Verification items for the finished model (mm, model axes). Face numbers are marked on the shaded views. Round coordinates to 2 decimals unless told otherwise and drop trailing zeros. Write each loop counter-clockwise with the first axis right and the second up, starting at its lowest first coordinate (ties: lowest second). Pieces come first, ordered by that corner, then holes. Notation, with made-up numbers: (0, 29.25) -> (19, 29.25) arc R27 cw to (19, 68.25) -> close; hole circle Ø8 at (89, 8.25). An arc over 180 degrees is marked (long way). Answer as a JSON object with one key per item and string values. Group by question number.
(1) Sectioned sample at A-A on z = 5.5. Record the cut outline in (x, y), and give its area (3 significant figures).
(2) Scan lines: L1, parallel to Z at x = -0.95, y = -0.2; L2, parallel to Z at x = 0.7, y = -2.4; L3, parallel to Y at x = 1.35, z = 1.25. Record each from-to range of solid material in increasing order. Write a range as from..to.
(3) Gauge pin test, flat ends, axial feed: pin 1 Ø2 at (y, z) = (-1.5, 14) entering from -X; pin 2 Ø2 at (y, z) = (-1, 7) entering from +X; pin 3 Ø0.9 at (x, z) = (0, 1) entering from -Y; pin 4 Ø1.6 at (x, y) = (0, 0) entering from -Z. Record the tip position at first contact, or that the pin passes through.
(4) Draft check along X on the marked faces 1, 2 and 3. Enter one of: released by +X, released by -X, zero draft, split by the parting line, or undercut.
```python
from build123d import *

# Parameters (mm, degrees)
F1_R     = 2.75
F1_R_2   = 1.5
F2_DEPTH = 2
F3_START = 1.5
F3_DEPTH = 0.5
F4_START = 2
F4_DEPTH = 15
F5_SIZE2 = 1.25
F5_SIZE  = 1.25
F6_R     = 0.25


# Not quite as in the source:
# - a feature names something its author has since deleted; it is built from what else it names


with BuildPart() as f2:
    # F1 (on Top) → F2 (new body)
    with BuildSketch(Plane.XY):
        Circle(F1_R)
        Circle(F1_R_2, mode=Mode.SUBTRACT)
        Circle(F1_R_2)
        Polygon((-0.5773502692, -1), (-1.1547005384, 0), (-0.5773502692, 1), (0.5773502692, 1), (1.1547005384, 0), (0.5773502692, -1), align=None, mode=Mode.SUBTRACT)
    extrude(amount=F2_DEPTH)

    # F1 (on Top) → F3 (join)
    with BuildSketch(Plane.XY.offset(F3_START)):
        Polygon((-0.5773502692, 1), (-1.1547005384, 0), (-0.5773502692, -1), (0.5773502692, -1), (1.1547005384, 0), (0.5773502692, 1), align=None)
    extrude(amount=F3_DEPTH)

    # F1 (on Top) → F4 (join)
    with BuildSketch(Plane.XY.offset(F4_START)):
        Circle(F1_R_2)
        Polygon((-0.5773502692, -1), (-1.1547005384, 0), (-0.5773502692, 1), (0.5773502692, 1), (1.1547005384, 0), (0.5773502692, -1), align=None, mode=Mode.SUBTRACT)
        Polygon((-0.5773502692, 1), (-1.1547005384, 0), (-0.5773502692, -1), (0.5773502692, -1), (1.1547005384, 0), (0.5773502692, 1), align=None)
    extrude(amount=F4_DEPTH)

    # F5
    f5_edges = [f2.edges().sort_by_distance(p)[0] for p in [
        (-2.75, 0, 0),
    ]]
    chamfer(f5_edges, length=F5_SIZE, length2=F5_SIZE2)

    # F6
    f6_edges = [f2.edges().sort_by_distance(p)[0] for p in [
        (-2.75, 0, 2),
        (-1.5, 0, 2),
        (-1.5, 0, 0),
        (-2.75, 0, 1.25),
    ]]
    fillet(f6_edges, radius=F6_R)


solid = f2.part
```
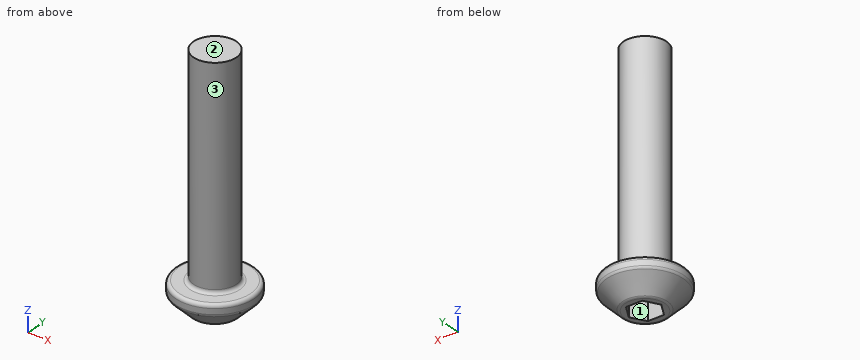
Computed values:
{
 "1": {"outline": "circle Ø3 at (0, 0)", "area": "7.07 mm2"},
 "2": {"L1": "1.5..17", "L2": "1..2", "L3": "-2.37..2.37"},
 "3": {"pin 1": "x = -1.41", "pin 2": "x = 1.5", "pin 3": "y = -2.75", "pin 4": "z = 1.5"},
 "4": {"face 1": "undercut", "face 2": "zero draft", "face 3": "split by the parting line"}
}
